Here's how the part is built. I have some questions about the finished solid (model axes, mm). Face numbers are marked on the shaded views. A direction names the side the tool comes from. Round coordinates to 2 decimals unless told otherwise and drop trailing zeros. Write each loop counter-clockwise with the first axis right and the second up, starting at its lowest first coordinate (ties: lowest second). Pieces come first, ordered by that corner, then holes. Notation, with made-up numbers: (61.5, 59.5) - (87.5, 59.5) arc R23 ccw to (87.5, 80.5) - close; hole circle Ø2 at (-38, 23.5). An arc over 180 degrees is marked (long way). Use one line per item in the form item = value. Start each with the question number.
1. Will these pins go through, and if not, where does the flat tip stop? pin 1 (1.8 mm diameter, centred on x = -15.5, z = -15, fed in from -Y); pin 2 (1.8 mm diameter, centred on x = 14.5, z = 15, fed in from -Y); pin 3 (0.5 mm diameter, centred on x = -2.5, z = 0, fed in from -Y); pin 4 (3 mm diameter, centred on x = -4, y = -15.5, fed in from -Z).
2. Which directions (+Z, -Z, +X, -X, +Y, -Y) give clear straight access to the entire face, cutting with the end or side of a thin tool? Please do the marked faces 1 and 2.
3. If I drill on line 1 along Z through (x, y) = (-15.5, 4.5); line 2 along X through (y, z) = (5, 15); line 3 along Y through (x, z) = (4, 17.5), over which ranges is the centre line in solid material (lowest first)?
4. I want a section at C-C, the plane x = 15.5. List the corners of the cut face in (y, z) for me.
5. I want a section at B-B, the plane z = 15.5. List the corners of the cut face in (x, y) for me, plus the area to 3 significant figures.
6. I want a section at D-D, the plane y = -20. List the corners of the cut face in (x, z) for me, plus the area to 3 significant figures.
7. I want a section at A-A, the plane y = 8.5. List the corners of the cut face in (x, z) for me, plus the area to 3 significant figures.
```python
from build123d import *

# Parameters (mm, degrees)
F0_R     = 1.75
F1_DEPTH = 42
F2_DEPTH = 2
F3_DEPTH = 24
F4_DEPTH = 10
F6_DEPTH = 18


with BuildPart() as f1:
    # F0 (on Front) → F1 (new body)
    with BuildSketch(Plane.XZ):
        Polygon((21.1, 21.1), (0, 21.1), (-21.1, 21.1), (-21.1, 0), (-21.1, -21.1), (0, -21.1), (21.1, -21.1), (21.1, 0), align=None)
        with Locations((-15.5, -15.5)):
            Circle(F0_R, mode=Mode.SUBTRACT)
        with Locations((15.5, -15.5)):
            Circle(F0_R, mode=Mode.SUBTRACT)
        with Locations((-15.5, 15.5)):
            Circle(F0_R, mode=Mode.SUBTRACT)
        with BuildLine():
            ThreePointArc((0, 11), (7.778175, 7.778175), (11, 0))
            ThreePointArc((11, 0), (7.778175, -7.778175), (0, -11))
            ThreePointArc((0, -11), (-7.778175, -7.778175), (-11, 0))
            ThreePointArc((-11, 0), (-7.778175, 7.778175), (0, 11))
        make_face(mode=Mode.SUBTRACT)
        with Locations((15.5, 15.5)):
            Circle(F0_R, mode=Mode.SUBTRACT)
        with BuildLine():
            ThreePointArc((0, -11), (7.778175, -7.778175), (11, 0))
            ThreePointArc((11, 0), (7.778175, 7.778175), (0, 11))
            ThreePointArc((0, 11), (-7.778175, 7.778175), (-11, 0))
            ThreePointArc((-11, 0), (-7.778175, -7.778175), (0, -11))
        make_face()
        with BuildLine():
            ThreePointArc((0, 2.5), (1.767767, 1.767767), (2.5, 0))
            ThreePointArc((2.5, 0), (1.767767, -1.767767), (0, -2.5))
            ThreePointArc((0, -2.5), (-1.767767, -1.767767), (-2.5, 0))
            ThreePointArc((-2.5, 0), (-1.767767, 1.767767), (0, 2.5))
        make_face(mode=Mode.SUBTRACT)
        with BuildLine():
            ThreePointArc((0, -2.5), (1.767767, -1.767767), (2.5, 0))
            ThreePointArc((2.5, 0), (1.767767, 1.767767), (0, 2.5))
            ThreePointArc((0, 2.5), (-1.767767, 1.767767), (-2.5, 0))
            ThreePointArc((-2.5, 0), (-1.767767, -1.767767), (0, -2.5))
        make_face()
        with Locations((15.5, 15.5)):
            Circle(F0_R)
        with Locations((-15.5, 15.5)):
            Circle(F0_R)
        with Locations((-15.5, -15.5)):
            Circle(F0_R)
        with Locations((15.5, -15.5)):
            Circle(F0_R)
    extrude(amount=-F1_DEPTH)

    # F0 (on Front) → F2 (join)
    with BuildSketch(Plane.XZ):
        with BuildLine():
            ThreePointArc((0, -11), (7.778175, -7.778175), (11, 0))
            ThreePointArc((11, 0), (7.778175, 7.778175), (0, 11))
            ThreePointArc((0, 11), (-7.778175, 7.778175), (-11, 0))
            ThreePointArc((-11, 0), (-7.778175, -7.778175), (0, -11))
        make_face()
        with BuildLine():
            ThreePointArc((0, 2.5), (1.767767, 1.767767), (2.5, 0))
            ThreePointArc((2.5, 0), (1.767767, -1.767767), (0, -2.5))
            ThreePointArc((0, -2.5), (-1.767767, -1.767767), (-2.5, 0))
            ThreePointArc((-2.5, 0), (-1.767767, 1.767767), (0, 2.5))
        make_face(mode=Mode.SUBTRACT)
    extrude(amount=F2_DEPTH)

    # F0 (on Front) → F3 (join)
    with BuildSketch(Plane.XZ):
        with BuildLine():
            ThreePointArc((0, -2.5), (1.767767, -1.767767), (2.5, 0))
            ThreePointArc((2.5, 0), (1.767767, 1.767767), (0, 2.5))
            ThreePointArc((0, 2.5), (-1.767767, 1.767767), (-2.5, 0))
            ThreePointArc((-2.5, 0), (-1.767767, -1.767767), (0, -2.5))
        make_face()
    extrude(amount=F3_DEPTH)

    # F0 (on Front) → F4 (cut)
    with BuildSketch(Plane.XZ):
        with Locations((-15.5, 15.5)):
            Circle(F0_R)
        with Locations((15.5, -15.5)):
            Circle(F0_R)
        with Locations((-15.5, -15.5)):
            Circle(F0_R)
        with Locations((15.5, 15.5)):
            Circle(F0_R)
    extrude(amount=-F4_DEPTH, mode=Mode.SUBTRACT)

    # F5 (on face) → F6 (cut)
    with BuildSketch(Plane.XZ.offset(24)):
        with BuildLine():
            Line((-2, 0), (-2, 1.5))
            ThreePointArc((-2, 1.5), (-2.5, 0), (-2, -1.5))
            Line((-2, -1.5), (-2, 0))
        make_face()
    extrude(amount=-F6_DEPTH, mode=Mode.SUBTRACT)


solid = f1.part
```
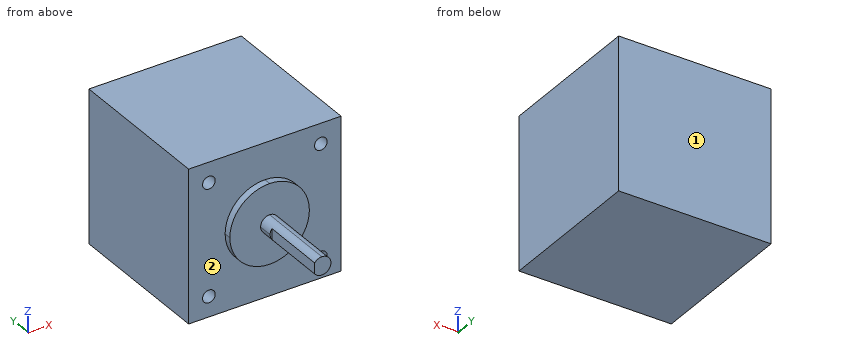
Model answer:
q1.pin_1 = 10
q1.pin_2 = 0
q1.pin_3 = -6
q1.pin_4 = through
q2.face_1 = +Z, -Z, +X, -X, +Y
q2.face_2 = -Y
q3.line_1 = -21.1 to -17.25, -13.75 to 13.75, 17.25 to 21.1
q3.line_2 = -21.1 to -17.18, -13.82 to 13.82, 17.18 to 21.1
q3.line_3 = 0 to 42
q4.outline = (0, -21.1) - (42, -21.1) - (42, 21.1) - (0, 21.1) - (0, 17.25) - (10, 17.25) - (10, 13.75) - (0, 13.75) - (0, -13.75) - (10, -13.75) - (10, -17.25) - (0, -17.25) - close
q5.outline = (-21.1, 0) - (-17.25, 0) - (-17.25, 10) - (-13.75, 10) - (-13.75, 0) - (13.75, 0) - (13.75, 10) - (17.25, 10) - (17.25, 0) - (21.1, 0) - (21.1, 42) - (-21.1, 42) - close
q5.area = 1,700 mm2
q6.outline = (-2, -1.5) arc R2.5 ccw (long way) to (-2, 1.5) - close
q6.area = 18.6 mm2
q7.outline = (-21.1, -21.1) - (21.1, -21.1) - (21.1, 21.1) - (-21.1, 21.1) - close; hole circle Ø3.5 at (-15.5, -15.5); hole circle Ø3.5 at (-15.5, 15.5); hole circle Ø3.5 at (15.5, -15.5); hole circle Ø3.5 at (15.5, 15.5)
q7.area = 1,740 mm2
